The listing builds one solid part. Answer for the finished solid, in the listing's coordinates (mm). Face numbers are marked on the shaded views. A direction names the side the tool comes from. Coordinates: 2 decimals unless noted, no trailing zeros. Loops run counter-clockwise (first coordinate to the right, second up) from the corner with the lowest first, then second, coordinate; pieces in that order, holes last. Notation, with made-up numbers: M 68.5,-8.5 L 112.5,-8.5 A15 cw 112.5,16.5 Z; hole C 18.5,-33.75 d4. An arc over 180 degrees is marked long. Answer as a JSON object with one key per item and string values. Group by question number.
1. A cutting plane is placed at C-C on x = -4.25. Give the vertices of the cut face in (y, z), and give its area (3 significant figures).
2. For the marked faces 1, 2 and 3, determine the directions among +Z, -Z, +X, -X, +Y, -Y from which every point of the face is accessible in a straight line to the end or side of a thin tool.
3. Determine the mould class of the marked faces 4, 5, 6 and 7 for opening direction X: released by +X, released by -X, zero draft, split by the parting line, or undercut.
4. Given pin 1 (2 mm diameter, centred on x = -14.5, z = 5, fed in from -Y); pin 2 (7.5 mm diameter, centred on x = -15, z = -1.5, fed in from -Y); pin 3 (1.5 mm diameter, centred on x = -2, y = 5, fed in from +Z); pin 4 (2 mm diameter, centred on y = 3, z = -2.5, fed in from -X), each flat-ended and moving along its own axis, determine where each tip first touches the part or whether it passes through.
5. A cutting plane is placed at A-A on z = 0. Give the vertices of the cut face in (x, y), and give its area (3 significant figures).
6. Straight lines are drawn through the part: L1, parallel to Z at x = -10, y = 4.25; L2, parallel to Y at x = -15.5, z = -1; L3, parallel to Z at x = -11.75, y = 2. For each, find the intervals that lie inside material, in ascending order.
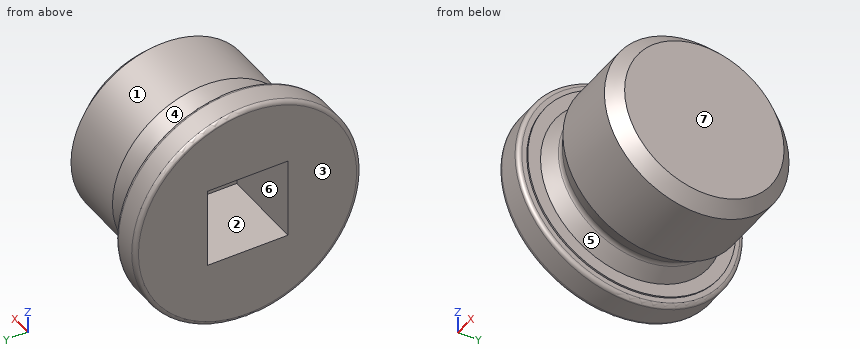
from build123d import *

# Parameters (mm, degrees)
SKETCH2_W          = 9.6
SKETCH2_H          = 9.6
CUT_EXTRUDE1_DEPTH = 10
FILLET1_R          = 0.5
SKETCH3_W          = 1.5
SKETCH3_H          = 2


with BuildPart() as part:
    # Sketch1 → Revolve1 (revolve)
    with BuildSketch(Plane.XY):
        with BuildLine():
            Line((0, 0), (0, 9.5))
            Line((0, 9.5), (-1.5, 11))
            Line((-1.5, 11), (-9.622450166, 11))
            Line((-9.622450166, 11), (-11.60187303, 9.857179677))
            ThreePointArc((-11.60187303, 9.857179677), (-12.000249041, 9.750001648), (-12.399056907, 9.855561401))
            Line((-12.399056907, 9.855561401), (-14.4, 11))
            Line((-14.4, 11), (-14.4, 13.5))
            Line((-14.4, 13.5), (-18, 13.5))
            Line((-18, 13.5), (-18, 0))
            Line((-18, 0), (0, 0))
        make_face()
    revolve(axis=Axis((0, 0, 0), (-1, 0, 0)))

    # Sketch2 → Cut-Extrude1 (cut)
    with BuildSketch(Plane.ZY.offset(18)):
        Rectangle(SKETCH2_W, SKETCH2_H)
    extrude(amount=-CUT_EXTRUDE1_DEPTH, mode=Mode.SUBTRACT)

    # Fillet1
    fillet1_edges = [part.edges().sort_by_distance(p)[0] for p in [
        (-14.4, -13.5, 0),
        (-18, -13.5, 0),
    ]]
    fillet(fillet1_edges, radius=FILLET1_R)

    # Sketch3 → Revolve2 (revolve)
    with BuildSketch(Plane.XY, mode=Mode.PRIVATE) as revolve2_sk:
        with Locations((-14.95, 11.4)):
            Rectangle(SKETCH3_W, SKETCH3_H)
    revolve(revolve2_sk.sketch.rotate(Axis((0, 0, 0), (-1, 0, 0)), 90), axis=Axis((0, 0, 0), (-1, 0, 0)))


solid = part.part
From the geometry:
{
 "1": {"outline": "C 0,0 d22", "area": "380 mm²"},
 "2": {"face 1": "+X", "face 2": "-X", "face 3": "+Z, -Z, -X, +Y, -Y"},
 "3": {"face 4": "undercut", "face 5": "undercut", "face 6": "zero draft", "face 7": "released by +X"},
 "4": {"pin 1": "stops at y = -12.87", "pin 2": "stops at y = -13.5", "pin 3": "stops at z = 10.15", "pin 4": "stops at x = -8"},
 "5": {"outline": "M -18,-13 A0.5 ccw -17.5,-13.5 L -14.9,-13.5 A0.5 ccw -14.4,-13 L -14.4,-12.4 L -14.2,-12.4 L -14.2,-10.89 L -12.4,-9.86 A0.8 cw -11.6,-9.86 L -9.62,-11 L -1.5,-11 L 0,-9.5 L 0,9.5 L -1.5,11 L -9.62,11 L -11.6,9.86 A0.8 cw -12.4,9.86 L -14.2,10.89 L -14.2,12.4 L -14.4,12.4 L -14.4,13 A0.5 ccw -14.9,13.5 L -17.5,13.5 A0.5 ccw -18,13 L -18,4.8 L -8,4.8 L -8,-4.8 L -18,-4.8 Z", "area": "310 mm²"},
 "6": {"L1": "z = -9.91 to -4.8, 4.8 to 9.91", "L2": "y = -13.46 to -4.8, 4.8 to 13.46", "L3": "z = -9.58 to -4.8, 4.8 to 9.58"}
}
